Study the drawing (mm; zero at the part's minimum x, y, z) and answer. Give positions to 0.01 mm unless a question says otherwise; leave off trailing zeros. Order: outer loops, then holes, each group sorted by start corner. A loop starts at its lowest first (then second) coordinate and runs counter-clockwise, first axis right, second up. Notation, with made-up numbers: (6, 60.25) - (51, 60.25) arc R18 ccw to (51, 66.25) - close; hole circle Ø8 at (11, -38.75). An arc over 180 degrees is marked (long way). Use CSV: the item, a comma, the result in double quotes.
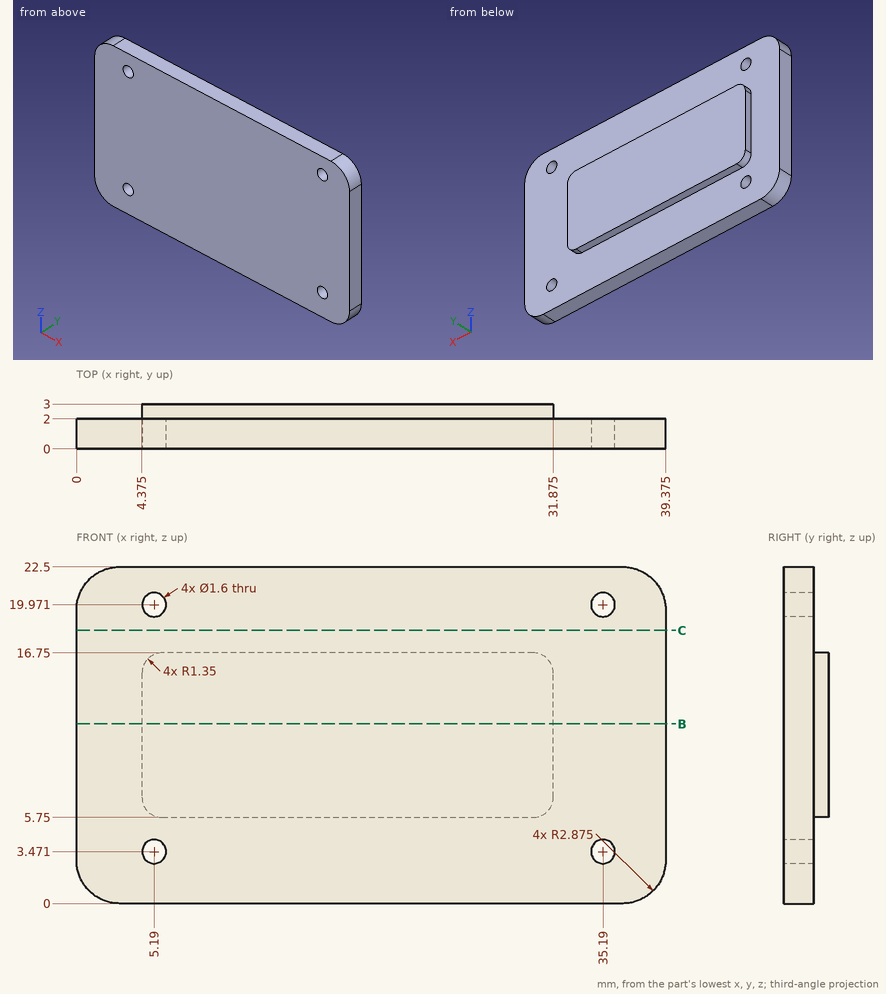
Item 1: Find the intervals of material crossed by line 1 along X through (y, z) = (0.4, 3.5) (1 decimal); line 2 along Z through (x, y) = (35, 0.3); line 3 along Y through (x, z) = (30, 20.5), in increasing order.
Taken from the geometry:
line 1,"0 to 4.4, 6 to 34.4, 36 to 39.4"
line 2,"0 to 2.69, 4.25 to 19.19, 20.75 to 22.5"
line 3,"0 to 2"
Item 2: The part is cut by section B-B (z = 12). Give the vertices of the cut face in (x, y) (1 decimal), and give its area (3 significant figures).
Taken from the geometry:
outline,"(0, 0) - (39.4, 0) - (39.4, 2) - (31.9, 2) - (31.9, 3) - (4.4, 3) - (4.4, 2) - (0, 2) - close"
area,"106 mm^2"
Item 3: The part is cut by section C-C (z = 18.25). Give the vertices of the cut face in (x, y) (1 decimal).
Taken from the geometry:
outline,"(0, 0) - (39.4, 0) - (39.4, 2) - (0, 2) - close"
Item 4: Each of these flat-tipped pins is pushed along its axis until it touches: pin 1 (5 mm diameter, centred on x = 5.5, z = 2.5, fed in from +Y); pin 2 (1.8 mm diameter, centred on x = 5.19, z = 19.97, fed in from -Y). Where does it stop, or does it pass through?
Taken from the geometry:
pin 1,"y = 2"
pin 2,"y = 0"
